Can you work these out from the model? Positions are in its coordinate system, mm. A direction names the side the tool comes from. Give positions to 0.01 mm unless a question says otherwise; leave off trailing zeros. Loops run counter-clockwise (first coordinate to the right, second up) from the corner with the lowest first, then second, coordinate; pieces in that order, holes last. Notation, with made-up numbers: (3.5, -8.5) - (37.5, -8.5) arc R9 cw to (37.5, -0.5) - close; hole circle Ø3 at (46, 87.5). An arc over 180 degrees is marked (long way). Answer in a Markdown table with one row per item.
Autodesk Inventor part; units mm, degrees
sketch "Sketch1" plane through (0, 0, 0) normal (0, 1, 0) x (-1, 0, 0)
  circle A0 centre (0, 0) radius 42.4
  circle A1 centre (0, 0) radius 52.4
  dimension "d0" = 84.8
  dimension "d1" = 10
extrude "Extrusion1" add sketch "Sketch1" along normal blind 14
fillet "Fillet1" radius 1 4 edges at (52.4, 14, 0) (42.4, 14, 0) (52.4, 0, 0) (42.4, 0, 0)
ref_plane "Work Plane1" through (52.4, 0, 0) normal (1, 0, 0) x (0, 1, 0)
sketch "Sketch2" plane through (52.4, 0, 0) normal (1, 0, 0) x (0, 1, 0)
  line L0 (0, 73.36) -> (0, -73.36)
  point P0 (0, 0)
  point P1 (7, 0)
  dimension "d5" = 7
hole "Hole1" at (52.4, 7, 0) direction (-1, 0, 0) diameter 3.4 end up to surface counterbore diameter 6.4 counterbore depth 2
pattern_circular "Circular Pattern1" count 2 over 360 about axis through (0, -10, 0) along (0, 1, 0) of "Hole1"
ref_plane "Work Plane7" through (0, 0, 52.4) normal (0, 0, 1) x (1, 0, 0)
sketch "Sketch8" plane through (0, 0, 52.4) normal (0, 0, 1) x (1, 0, 0)
  line L0 (-73.36, 0) -> (73.36, 0)
  point P0 (0, 0)
  point P1 (0, 7)
  dimension "d53" = 7
hole "Hole5" at (0, 7, 52.4) direction (0, 0, -1) diameter 4 depth 5.8
pattern_circular "Circular Pattern4" count 2 over 360 about axis through (0, -10, 0) along (0, 1, 0) of "Hole5"
properties part number "o-ring" material "ABS Plastic"
Q1. Imagine slicing it at B-B, the plane z = 0. Count the separate pieces of the cut face and the enclosed holes in it, and give its area (3 significant figures).
Checked values:
| item | result |
|---|---|
| separate pieces | 4 |
| enclosed holes | 0 |
| area | 198 mm² |
Q2. On a 3-axis mill with a long thin cutter (end or side, diameter ignored), from which of +Z, -Z, +X, -X, +Y, -Y can I reach the whole of each face in a straight line? I mean faces 4 (the face through (0, 7, -46.6)), 5 (the face through (50.4, 8.4, -1.4)), 6 (the face through (0, 9, 49)). Say none if no direction works.
Checked values:
| item | result |
|---|---|
| face 4 | -Z |
| face 5 | +X |
| face 6 | +Z |
Q3. If I drill on line 1 (Y direction, x = 0, z = 50); line 2 (X direction, y = 10.75, z = 0); line 3 (X direction, y = 5.5, z = -2), over which ranges is the centre line in solid material (lowest first)? Write a range as [from, to].
Checked values:
| item | result |
|---|---|
| line 1 | y = [0, 5], [9, 14] |
| line 2 | x = [-52.4, -42.4], [42.4, 52.4] |
| line 3 | x = [-50.4, -42.35], [42.35, 50.4] |
Q4. Imagine slicing it at A-A, the plane x = 0. Write out the boundary of the cut face in (y, z).
Checked values:
| item | result |
|---|---|
| outline | (0, -51.4) arc R1 ccw to (1, -52.4) - (5, -52.4) - (5, -46.6) - (9, -46.6) - (9, -52.4) - (13, -52.4) arc R1 ccw to (14, -51.4) - (14, -43.4) arc R1 ccw to (13, -42.4) - (1, -42.4) arc R1 ccw to (0, -43.4) - close; (0, 43.4) arc R1 ccw to (1, 42.4) - (13, 42.4) arc R1 ccw to (14, 43.4) - (14, 51.4) arc R1 ccw to (13, 52.4) - (9, 52.4) - (9, 46.6) - (5, 46.6) - (5, 52.4) - (1, 52.4) arc R1 ccw to (0, 51.4) - close |
Q5. If we mould it in two halves opening along Z, with no side actions, what happens to faces 1 (the face through (-50.4, 8.4, -1.4)), 2 (the face through (0, 9, -49)), 3 (the face through (-49.98, 6.92, -15.74))? For each: released by +Z, released by -Z, zero draft, split by the parting line, or undercut.
Checked values:
| item | result |
|---|---|
| face 1 | undercut |
| face 2 | zero draft |
| face 3 | split by the parting line |
Q6. For pin 1 (8 mm diameter, centred on y = 10, z = 30, fed in from +X); pin 2 (2 mm diameter, centred on x = 0, y = 7, fed in from +Z); pin 3 (2 mm diameter, centred on x = 3, y = 11, fed in from -Z), each with a flat end and sliding along its axis, tell me the tip position at first contact or that it passes through.
Checked values:
| item | result |
|---|---|
| pin 1 | stops at x = 45.49 |
| pin 2 | stops at z = 46.6 |
| pin 3 | stops at z = -52.36 |
